Input: dimensioned drawing with shaded views. Units: mm. Origin: part minimum x, y, z. Give positions to 0.01 mm unless a question says otherwise; leave off trailing zeros. Write each loop counter-clockwise with the first axis right and the second up, starting at its lowest first coordinate (ties: lowest second). Pieces come first, ordered by that corner, then holes. Notation, with made-up numbers: (0.5, 78) -> (54.5, 78) arc R11 cw to (54.5, 88) -> close; hole circle Ø7 at (42.5, -34.5). An arc over 180 degrees is marked (long way). Answer as a JSON object with one key per item and string values. Group by question number.
(1) Contact query for flat-ended pins moving along their axis: pin 1 Ø1 at (y, z) = (1, 1.5) entering from -X; pin 2 Ø1 at (y, z) = (3, 1.5) entering from -X. Output: stop coordinate, or through.
(2) Draft query along X for the marked faces 1, 2 and 3. Return one class per face: +X half, -X half, draft (parallel to the pull), parting line (faces both ways), or undercut.
(3) Section query A-A on z = 3.45. Output: boundary loops of the cut face in (x, y) (1 decimal).
(4) Material intervals for probe 1 along Y at (x, z) = (2.4, 3.8); probe 2 along Y at (x, z) = (2.9, 0.5) (1 decimal), sorted ascending.
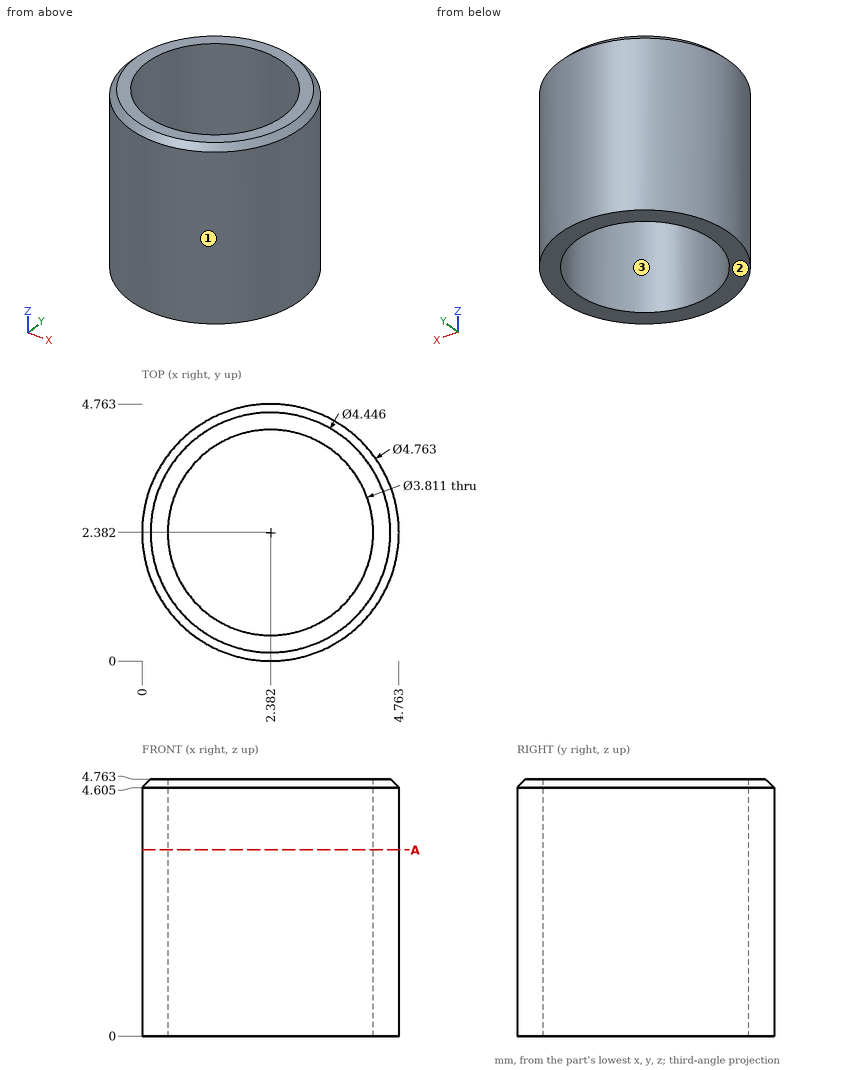
Answer list:
{
 "1": {"pin 1": "x = 0.17", "pin 2": "x = 0"},
 "2": {"face 1": "parting line", "face 2": "draft", "face 3": "undercut"},
 "3": {"outline": "circle Ø4.8 at (2.4, 2.4); hole circle Ø3.8 at (2.4, 2.4)"},
 "4": {"probe 1": "0 to 0.48, 4.29 to 4.76", "probe 2": "0.1 to 0.5, 4.2 to 4.7"}
}
